Could you check a few things on this model? Use its own coordinates, in mm. A direction names the side the tool comes from. Coordinates: 2 decimals unless noted, no trailing zeros. Loops run counter-clockwise (first coordinate to the right, second up) from the corner with the lowest first, then second, coordinate; pieces in that order, holes last. Notation, with made-up numbers: (28.5, 63) - (59.5, 63) arc R20 ccw to (59.5, 92) - close; hole circle Ø10 at (0.5, 19). An arc over 180 degrees is marked (long way). One line per item, written item: value. Start each with the question number.
(1) On a 3-axis mill with a long thin cutter (end or side, diameter ignored), from which of +Z, -Z, +X, -X, +Y, -Y can I reach the whole of each face in a straight line? I mean faces 4 (the face through (-17, -2, -7.24)), 5 (the face through (6.6, 11.7, 0.875)), 6 (the face through (-21.46, -2, -2)), 7 (the face through (14, -2, -5.34)), 8 (the face through (12.55, -3.94, 5.69)). Say none if no direction works.
(2) If we section it at A-A on y = 4.75: Write out the boundary of the cut face in (x, z), then the cut area to 3 significant figures.
(3) If we section it at B-B on z = 7.69: Write out the boundary of the cut face in (x, y), then the cut area to 3 significant figures.
(4) If we section it at C-C on y = -5.5: Write out the boundary of the cut face in (x, z) (3 decimals).
(5) I'm going to push flat-ended pins straight in: P1, Ø1.5, axis at x = -21.5, y = -4.5, coming from the +Z side; P2, Ø2, axis at y = 2.5, z = 8, coming from the +X side; P3, Ø3.5, axis at y = -2.5, z = -2.5, coming from the +X side. Where does each tip first touch, or does it pass through?
(6) If we mould it in two halves opening along X, with no side actions, what happens to faces 1 (the face through (19.29, 17.14, -1.08)), 2 (the face through (-17, -2, 3.76)), 3 (the face through (20.925, 10.788, -1.153))? For each: pulls with the +X half, pulls with the -X half, needs draft (parallel to the pull), parting line crosses it, or undercut.
(7) If I drill on line 1 along X through (y, z) = (8.5, 2.75); line 2 along Z through (x, y) = (9, 14); line 3 along Y through (x, z) = (-5, -6.75), over which ranges is the centre line in solid material (lowest first)? Write a range as from..to.
(8) If we section it at D-D on x = -8.5: Write out the boundary of the cut face in (y, z), then the cut area to 3 significant figures.
```python
from build123d import *

# Parameters (mm, degrees)
SKETCH1_W                = 58.2
SKETCH1_H                = 20.22
BOSS_EXTRUDE1_DEPTH      = 1
BOSS_EXTRUDE2_DEPTH      = 14
BOSS_EXTRUDE2_DEPTH_BACK = 5.2
SKETCH2_W                = 9.67
SKETCH2_H                = 11
SKETCH3_R                = 2.42
BOSS_EXTRUDE3_DEPTH      = 11
BOSS_EXTRUDE4_DEPTH      = 13.4
BOSS_EXTRUDE4_DEPTH_BACK = 4.3
SKETCH4_W                = 13.2
SKETCH4_H                = 8.43
SKETCH7_W                = 11.57
SKETCH7_H                = 6.8
BOSS_EXTRUDE5_DEPTH      = 3.35
CUT_EXTRUDE1_DEPTH       = 38.095225097
CUT_EXTRUDE1_DEPTH_BACK  = 38.095225097
EXTRUDE_THIN2_DEPTH      = 2
SKETCH10_R               = 0.775
BOSS_EXTRUDE6_DEPTH      = 8
SKETCH12_W               = 1.5
SKETCH12_H               = 1.25
BOSS_EXTRUDE7_DEPTH      = 1


with BuildPart() as part:
    # Sketch1 → Boss-Extrude1 (new body)
    with BuildSketch(Plane(origin=(0, 0, 0), x_dir=(1, 0, 0), z_dir=(0, 1, 0))):
        Rectangle(SKETCH1_W, SKETCH1_H)
    extrude(amount=BOSS_EXTRUDE1_DEPTH)

    # Sketch2 → Boss-Extrude2 (add, two sides: drawn at the far end of the back side and taken through both)
    with BuildSketch(Plane(origin=(0, 1, 0), x_dir=(1, 0, 0), z_dir=(0, 1, 0)).offset(-BOSS_EXTRUDE2_DEPTH_BACK)):
        with Locations((-16.625, 1.74)):
            Rectangle(SKETCH2_W, SKETCH2_H)
    extrude(amount=BOSS_EXTRUDE2_DEPTH + BOSS_EXTRUDE2_DEPTH_BACK)

    # Sketch3 → Boss-Extrude3 (add)
    with BuildSketch(Plane(origin=(0, 1, 0), x_dir=(1, 0, 0), z_dir=(0, 1, 0))):
        with Locations(Location((1.57, -7.69, 0), (0, 0, 270))):
            Circle(SKETCH3_R)
    extrude(amount=BOSS_EXTRUDE3_DEPTH)

    # Sketch4 → Boss-Extrude4 (add, two sides: drawn at the far end of the back side and taken through both)
    with BuildSketch(Plane(origin=(0, 1, 0), x_dir=(1, 0, 0), z_dir=(0, 1, 0)).offset(-BOSS_EXTRUDE4_DEPTH_BACK)):
        with Locations((14.04, 1.125)):
            Rectangle(SKETCH4_W, SKETCH4_H)
    extrude(amount=BOSS_EXTRUDE4_DEPTH + BOSS_EXTRUDE4_DEPTH_BACK)

    # Sweep1: sweep along a path in Sketch6
    with BuildLine(Plane(origin=(0, 14.4, 0), x_dir=(1, 0, 0), z_dir=(0, 1, 0))) as sweep1_path:
        Line((7.44, 5.34), (7.44, -3.09))
        Line((7.44, -3.09), (20.64, -3.09))
        Line((20.64, -3.09), (20.64, 5.34))
        Line((20.64, 5.34), (7.44, 5.34))
    # Sketch5 → Sweep1 (sweep)
    with BuildSketch(Plane.ZY.offset(-7.44)):
        Polygon((3.09, 14.4), (4.09, 14.4), (4.09, 15.4), (2.93, 16.25), (2.275, 16.25), (2.275, 14.4), align=None)
    sweep(path=sweep1_path.line, transition=Transition.RIGHT)

    # Sketch7 → Boss-Extrude5 (add)
    with BuildSketch(Plane(origin=(0, 14.4, 0), x_dir=(1, 0, 0), z_dir=(0, 1, 0))):
        with Locations((14.04, 1.125)):
            Rectangle(SKETCH7_W, SKETCH7_H)
    extrude(amount=BOSS_EXTRUDE5_DEPTH)

    # Sketch8 → Cut-Extrude1 (cut, two sides: drawn at the far end of the back side and taken through both)
    with BuildSketch(Plane(origin=(0, 0, -4.525), x_dir=(-1, 0, 0), z_dir=(0, 0, -1)).offset(-CUT_EXTRUDE1_DEPTH_BACK)):
        with BuildLine():
            ThreePointArc((-19.825, 16.25), (-19.277156121, 17.153507794), (-18.405, 17.75))
            Line((-18.405, 17.75), (-19.825, 17.75))
            Line((-19.825, 17.75), (-19.825, 16.25))
        make_face()
        with BuildLine():
            ThreePointArc((-18.405, 17.75), (-16.236771779, 17.375407367), (-14.04, 17.25))
            Line((-14.04, 17.25), (-14.04, 17.75))
            Line((-14.04, 17.75), (-18.405, 17.75))
        make_face()
        with BuildLine():
            Line((-14.04, 17.75), (-14.04, 17.25))
            ThreePointArc((-14.04, 17.25), (-11.843228221, 17.375407367), (-9.675, 17.75))
            Line((-9.675, 17.75), (-14.04, 17.75))
        make_face()
        with BuildLine():
            Line((-8.255, 17.75), (-9.675, 17.75))
            ThreePointArc((-9.675, 17.75), (-8.802843879, 17.153507794), (-8.255, 16.25))
            Line((-8.255, 16.25), (-8.255, 17.75))
        make_face()
    extrude(amount=CUT_EXTRUDE1_DEPTH + CUT_EXTRUDE1_DEPTH_BACK, mode=Mode.SUBTRACT)

    # Sketch9 → Extrude-Thin2 (add, symmetric)
    with BuildSketch(Plane(origin=(0, 0, -1.125), x_dir=(-1, 0, 0), z_dir=(0, 0, -1))):
        Polygon((-20.988853725, 14.920998164), (-21.1, 14.4), (-21.74, 11.4), (-19.788926462, 6.965741958), (-19.331268945, 7.167111265), (-21.217317359, 11.453584933), (-20.611003582, 14.295680764), (-20.499857307, 14.816678928), align=None)
    extrude_thin2 = extrude(amount=EXTRUDE_THIN2_DEPTH, both=True)

    # Mirror1: Extrude-Thin2 across plane
    add(extrude_thin2.mirror(Plane(origin=(14.04, 0, 0), x_dir=(0, 0, 1), z_dir=(1, 0, 0))))

    # Sketch10 → Boss-Extrude6 (add)
    with BuildSketch(Plane.XZ):
        with Locations(Location((-10.1, 6.11, 0), (0, 0, 270))):
            Circle(SKETCH10_R)
        with Locations(Location((11.9, 6.11, 0), (0, 0, 270))):
            Circle(SKETCH10_R)
    extrude(amount=BOSS_EXTRUDE6_DEPTH)

    # Sketch12 → Boss-Extrude7 (add)
    with BuildSketch(Plane(origin=(0, 1, 0), x_dir=(1, 0, 0), z_dir=(0, 1, 0))):
        with Locations((-17.29, 8.885)):
            Rectangle(SKETCH12_W, SKETCH12_H)
        with Locations((-11.265, 8.885)):
            Rectangle(SKETCH12_W, SKETCH12_H)
        with Locations((-5.24, 8.885)):
            Rectangle(SKETCH12_W, SKETCH12_H)
        with Locations((0.785, 8.885)):
            Rectangle(SKETCH12_W, SKETCH12_H)
        with Locations((6.81, 8.885)):
            Rectangle(SKETCH12_W, SKETCH12_H)
    extrude(amount=BOSS_EXTRUDE7_DEPTH)


solid = part.part
```
Values:
1. face 4: -Z, +X, -X, -Y
1. face 5: +Z
1. face 6: +Z, -Z, -X, -Y
1. face 7: -Z, +X, -Y
1. face 8: -Y
2. outline: (-21.46, -7.24) - (-11.79, -7.24) - (-11.79, 3.76) - (-21.46, 3.76) - close; circle Ø4.84 at (1.57, 7.69); (7.44, -5.34) - (20.64, -5.34) - (20.64, 3.09) - (7.44, 3.09) - close
2. area: 236 mm2
3. outline: (-29.1, 0) - (29.1, 0) - (29.1, 1) - (3.99, 1) - (3.99, 12) - (-0.85, 12) - (-0.85, 1) - (-29.1, 1) - close
3. area: 111 mm2
4. outline: circle Ø1.55 at (-10.1, 6.11); circle Ø1.55 at (11.9, 6.11)
5. P1: stops at z = 3.76
5. P2: stops at x = 3.99
5. P3: stops at x = 20.64
6. face 1: pulls with the +X half
6. face 2: needs draft
6. face 3: undercut
7. line 1: x = -21.46..-11.79, 7.44..20.64
7. line 2: z = -5.34..3.09
7. line 3: y = 0..1
8. outline: (0, -10.11) - (1, -10.11) - (1, 10.11) - (0, 10.11) - close
8. area: 20.2 mm2
